```python
from build123d import *

# Parameters (mm, degrees)
SKETCH_1_R          = 185
SKETCH_1_R_2        = 1.5
EXTRUDE_1_DEPTH     = 3
SKETCH_2_R          = 2
CUT_EXTRUDE_1_DEPTH = 10


with BuildPart() as part:
    # 草图1 → 凸台-拉伸1 (new body)
    with BuildSketch(Plane.XY):
        Circle(SKETCH_1_R)
        with Locations((-120, 120)):
            Circle(SKETCH_1_R_2, mode=Mode.SUBTRACT)
        with Locations((120, 120)):
            Circle(SKETCH_1_R_2, mode=Mode.SUBTRACT)
        with Locations((120, -120)):
            Circle(SKETCH_1_R_2, mode=Mode.SUBTRACT)
        with Locations((-120, -120)):
            Circle(SKETCH_1_R_2, mode=Mode.SUBTRACT)
        with BuildLine():
            Line((-102.5, -75), (-102.5, 75))
            ThreePointArc((-102.5, 75), (-97.5, 80), (-92.5, 75))
            Line((-92.5, 75), (-92.5, -75))
            ThreePointArc((-92.5, -75), (-97.5, -80), (-102.5, -75))
        make_face(mode=Mode.SUBTRACT)
        with BuildLine():
            Line((147.5, -75), (147.5, 75))
            ThreePointArc((147.5, 75), (142.5, 80), (137.5, 75))
            Line((137.5, 75), (137.5, -75))
            ThreePointArc((137.5, -75), (142.5, -80), (147.5, -75))
        make_face(mode=Mode.SUBTRACT)
        with BuildLine():
            Line((-147.5, -75), (-147.5, 75))
            ThreePointArc((-147.5, 75), (-142.5, 80), (-137.5, 75))
            Line((-137.5, 75), (-137.5, -75))
            ThreePointArc((-137.5, -75), (-142.5, -80), (-147.5, -75))
        make_face(mode=Mode.SUBTRACT)
        with BuildLine():
            Line((-75, -102.5), (75, -102.5))
            ThreePointArc((75, -102.5), (80, -97.5), (75, -92.5))
            Line((75, -92.5), (-75, -92.5))
            ThreePointArc((-75, -92.5), (-80, -97.5), (-75, -102.5))
        make_face(mode=Mode.SUBTRACT)
        with BuildLine():
            Line((-75, 147.5), (75, 147.5))
            ThreePointArc((75, 147.5), (80, 142.5), (75, 137.5))
            Line((75, 137.5), (-75, 137.5))
            ThreePointArc((-75, 137.5), (-80, 142.5), (-75, 147.5))
        make_face(mode=Mode.SUBTRACT)
        with BuildLine():
            Line((102.5, -75), (102.5, 75))
            ThreePointArc((102.5, 75), (97.5, 80), (92.5, 75))
            Line((92.5, 75), (92.5, -75))
            ThreePointArc((92.5, -75), (97.5, -80), (102.5, -75))
        make_face(mode=Mode.SUBTRACT)
    extrude(amount=EXTRUDE_1_DEPTH)

    # 草图2 → 切除-拉伸1 (cut)
    with BuildSketch(Plane.XY.offset(3)):
        with Locations((0, 49.5)):
            Circle(SKETCH_2_R)
        with Locations((0, -49.5)):
            Circle(SKETCH_2_R)
        with Locations((49.5, 0)):
            Circle(SKETCH_2_R)
        with Locations((-49.5, 0)):
            Circle(SKETCH_2_R)
        with Locations((60, 100)):
            Circle(SKETCH_2_R)
        with Locations((-60, 100)):
            Circle(SKETCH_2_R)
    extrude(amount=-CUT_EXTRUDE_1_DEPTH, mode=Mode.SUBTRACT)


solid = part.part
```
Source: CAD feature listing. Evaluate the final solid. Frame: model axes, mm. Give positions to 0.01 mm unless a question says otherwise; leave off trailing zeros. Order: outer loops, then holes, each group sorted by start corner. A loop starts at its lowest first (then second) coordinate and runs counter-clockwise, first axis right, second up. Notation, with made-up numbers: (-28, -10.75) -> (11, -10.75) arc R10 cw to (11, 4.25) -> close; hole circle Ø4 at (-18, 49). An arc over 180 degrees is marked (long way). Use a Markdown table: item, result.
Q1. Section C-C (z = 2.5). State how many separate pieces and enclosed holes the cut face has, and give its area (3 significant figures).
A:
| item | result |
|---|---|
| separate pieces | 1 |
| enclosed holes | 16 |
| area | 97,900 mm^2 |
Q2. Section D-D (y = -87). Return the cut outline in (x, z).
A:
| item | result |
|---|---|
| outline | (-163.27, 0) -> (163.27, 0) -> (163.27, 3) -> (-163.27, 3) -> close |
Q3. Section B-B (x = 43). Return the cut outline in (y, z), and give its area (3 significant figures).
A:
| item | result |
|---|---|
| outline | (-179.93, 0) -> (-102.5, 0) -> (-102.5, 3) -> (-179.93, 3) -> close; (-92.5, 0) -> (137.5, 0) -> (137.5, 3) -> (-92.5, 3) -> close; (147.5, 0) -> (179.93, 0) -> (179.93, 3) -> (147.5, 3) -> close |
| area | 1,020 mm^2 |
Q4. First-contact query: P1, Ø0.9, axis at x = 22.5, z = 2, coming from the +Y side; P2, Ø1, axis at y = -49.5, z = 2, coming from the +X side; P3, Ø1.5, axis at x = -17.5, z = 2, coming from the +Y side; P4, Ø2.5, axis at x = -120, y = 120, coming from the +Z side. Flat tips, straight axial feed; report the tip coordinate or a pass-through.
A:
| item | result |
|---|---|
| P1 | y = 183.68 |
| P2 | x = 178.39 |
| P3 | y = 184.24 |
| P4 | through |
Q5. Section A-A (y = 30.5). Return the cut outline in (x, z).
A:
| item | result |
|---|---|
| outline | (-182.47, 0) -> (-147.5, 0) -> (-147.5, 3) -> (-182.47, 3) -> close; (-137.5, 0) -> (-102.5, 0) -> (-102.5, 3) -> (-137.5, 3) -> close; (-92.5, 0) -> (92.5, 0) -> (92.5, 3) -> (-92.5, 3) -> close; (102.5, 0) -> (137.5, 0) -> (137.5, 3) -> (102.5, 3) -> close; (147.5, 0) -> (182.47, 0) -> (182.47, 3) -> (147.5, 3) -> close |
Q6. Material intervals for line 1 (Y direction, x = -66, z = 2.75); line 2 (Y direction, x = 43, z = 0.5); line 3 (X direction, y = 45.5, z = 2.6), sorted ascending. Write a range as [from, to].
A:
| item | result |
|---|---|
| line 1 | [-172.83, -102.5], [-92.5, 137.5], [147.5, 172.83] |
| line 2 | [-179.93, -102.5], [-92.5, 137.5], [147.5, 179.93] |
| line 3 | [-179.32, -147.5], [-137.5, -102.5], [-92.5, 92.5], [102.5, 137.5], [147.5, 179.32] |
